Could you check a few things on this model? Use its own coordinates, in mm. Face numbers are marked on the shaded views. A direction names the side the tool comes from. Give positions to 0.01 mm unless a question says otherwise; leave off trailing zeros. Write each loop counter-clockwise with the first axis right and the second up, starting at its lowest first coordinate (ties: lowest second). Pieces come first, ordered by that corner, then holes. Notation, with made-up numbers: (-24.75, 65) -> (-15.75, 65) arc R15 ccw to (-15.75, 94) -> close; hole circle Ø4 at (-25.5, 5.25). An arc over 180 degrees is marked (long way). One line per question, with ' | ' between items.
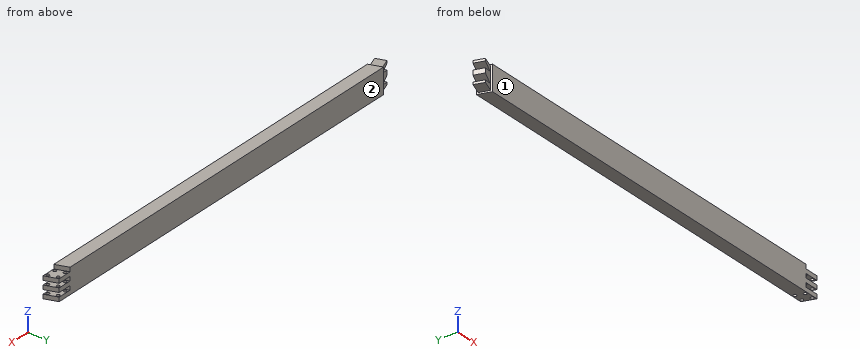
from build123d import *

# Parameters (mm, degrees)
F1_DEPTH  = 50.8
F2_W      = 27.051
F2_H      = 8.4666666667
F5_W      = 20.6801154209
F5_H      = 44.45
F8_DEPTH  = 31.6481136174
F9_R      = 3.175
F10_DEPTH = 42.3343333333


with BuildPart() as f1:
    # F0 (on Top) → F1 (new body)
    with BuildSketch(Plane.XY):
        Polygon((396.206887363, 12.7), (-414.6965752637, 12.7), (-405.4517313133, -12.7), (405.4517313133, -12.7), align=None)
    extrude(amount=F1_DEPTH)

    # F3: sweep along a path in F3_path
    with BuildLine(Plane(origin=(405.4517313133, -12.7, 50.8), x_dir=(0.3420201433, -0.9396926208, 0), z_dir=(0.9396926208, 0.3420201433, 0))) as f3_path:
        Line((0, 0), (-27.0301154209, 0))
    # F2 (on face) → F3 (sweep, cut)
    with BuildSketch(Plane(origin=(0, 12.7, 0), x_dir=(-1, 0, 0), z_dir=(0, 1, 0))):
        with Locations((-382.681387363, 12.7)):
            Rectangle(F2_W, F2_H)
        with Locations((-382.681387363, 29.6333333333)):
            Rectangle(F2_W, F2_H)
        with Locations((-382.681387363, 46.5666666667)):
            Rectangle(F2_W, F2_H)
    sweep(path=f3_path.line, mode=Mode.SUBTRACT)

    # F6: sweep along a path in F4
    with BuildLine(Plane.XY.offset(50.8)) as f6_path:
        Line((-405.4517313133, -12.7), (-429.3199238813, -21.3873116405))
    # F5 (on face) → F6 (sweep)
    with BuildSketch(Plane(origin=(-362.1045898409, -131.7952923933, 0), x_dir=(0.3420201433, -0.9396926208, 0), z_dir=(-0.9396926208, -0.3420201433, 0))):
        with Locations((-140.2536206819, 25.4)):
            Rectangle(F5_W, F5_H)
    sweep(path=f6_path.line)

    # F7 (on face) → F8 (cut, through all)
    with BuildSketch(Plane(origin=(-44.4330554274, 122.0788164643, 0), x_dir=(0.9396926208, 0.3420201433, 0), z_dir=(0.3420201433, -0.9396926208, 0))):
        Polygon((-388.5186558202, 36.5125), (-410.7436558202, 42.8625), (-410.7436558202, 30.1625), align=None)
        Polygon((-388.5186558202, 14.2875), (-410.7436558202, 20.6375), (-410.7436558202, 7.9375), align=None)
    extrude(amount=-F8_DEPTH, mode=Mode.SUBTRACT)

    # F9 (on face) → F10 (cut, through all)
    with BuildSketch(Plane.XY.offset(42.3333333333)):
        with Locations((393.0055384983, 8.128)):
            Circle(F9_R)
        with Locations((375.6853800498, 8.128)):
            Circle(F9_R)
        with Locations((381.602080178, -8.128)):
            Circle(F9_R)
        with Locations((398.9222386265, -8.128)):
            Circle(F9_R)
    extrude(amount=-F10_DEPTH, mode=Mode.SUBTRACT)


solid = f1.part
Q1. On a 3-axis mill with a long thin cutter (end or side, diameter ignored), from which of +Z, -Z, +X, -X, +Y, -Y can I reach the whole of each face in a straight line? I mean the marked faces 1 and 2. Say none if no direction works.
Answer below:
face 1: +Z, -Z, +X, -Y | face 2: +Z, -Z, +X, -X, +Y
Q2. If I drill on line 1 along Y through (x, z) = (220, 14.5); line 2 along X through (y, z) = (-5, 44), over which ranges is the centre line in solid material (lowest first)?
Answer below:
line 1: y = -12.7 to 12.7 | line 2: x = -435.28 to 375.6
Q3. Will these pins go through, and if not, where does the flat tip stop? pin 1 (7.5 mm diameter, centred on x = 398.92, y = -8.13, fed in from +Z); pin 2 (5 mm diameter, centred on x = 266.5, y = 8.5, fed in from -Z); pin 3 (5 mm diameter, centred on x = -105, z = 5.5, fed in from -Y); pin 4 (4 mm diameter, centred on y = -2, z = 16.5, fed in from +X).
Answer below:
pin 1: stops at z = 42.33 | pin 2: stops at z = 0 | pin 3: stops at y = -12.7 | pin 4: stops at x = 402.27
Q4. Imagine slicing it at A-A on x = 169. Please give me the cut outline in (y, z).
Answer below:
outline: (-12.7, 0) -> (12.7, 0) -> (12.7, 50.8) -> (-12.7, 50.8) -> close
